Build history of the part. All positions in model axes, mm. Face numbers are marked on the shaded views. A direction names the side the tool comes from. Round coordinates to 2 decimals unless told otherwise and drop trailing zeros. Loops run counter-clockwise (first coordinate to the right, second up) from the corner with the lowest first, then second, coordinate; pieces in that order, holes last. Notation, with made-up numbers: M 31,58 L 46,58 A25 ccw 46,79 Z; hole C -36.75,87.25 d9. An arc over 180 degrees is marked long. Use one line per item in the form item = value. Start each with the question number.
Autodesk Inventor part; units mm, degrees
ref_plane "Startebene" through (0, 0, 0) normal (0, 0, 1) x (1, 0, 0)
ref_plane "Endebene" through (0, 0, 160) normal (0, 0, 1) x (1, 0, 0)
ref_plane "YZ Plane" through (0, 0, 0) normal (1, 0, 0) x (0, 1, 0)
ref_plane "Startebene" through (0, 0, 0) normal (0, 0, 1) x (1, 0, 0)
ref_plane "Endebene" through (0, 0, 160) normal (0, 0, 1) x (1, 0, 0)
sketch "Skizze" plane through (0, 0, 0) normal (0, 0, 1) x (1, 0, 0)
  line L0 (-30, -38) -> (-30, 38)
  line L1 (-18, 50) -> (18, 50)
  line L2 (30, 38) -> (30, -38)
  line L3 (18, -50) -> (-18, -50)
  arc A0 (-30, -38) -> (-18, -50) centre (-18, -38) ccw
  arc A1 (-18, 50) -> (-30, 38) centre (-18, 38) ccw
  arc A2 (30, 38) -> (18, 50) centre (18, 38) ccw
  arc A3 (18, -50) -> (30, -38) centre (18, -38) ccw
  line L4 (-14, 42) -> (14, 42)
  line L5 (22, 34) -> (22, -34)
  line L6 (14, -42) -> (-14, -42)
  line L7 (-22, -34) -> (-22, 34)
  line L8 (0, 73.4794) -> (0, -73.4794) construction
  line L9 (-45.4794, 0) -> (45.4794, 0) construction
  arc A4 (-22, -34) -> (-14, -42) centre (-14, -34) ccw
  arc A5 (-14, 42) -> (-22, 34) centre (-14, 34) ccw
  arc A6 (22, 34) -> (14, 42) centre (14, 34) ccw
  arc A7 (14, -42) -> (22, -34) centre (14, -34) ccw
  dimension "d7" = 12
  dimension "d10" = 100
  dimension "d11" = 60
  dimension "d12" = 8
  dimension "d15" = 50
  dimension "d16" = 30
  dimension "d19" = 8
  dimension "d20" = 8
extrude "Körper" add sketch "Skizze" along normal up to surface (160 mm away) from surface at 0
sketch "Sketch3" plane through (0, 0, 0) normal (0, 0, 1) x (1, 0, 0)
  line L0 (0, 0) -> (10, 0)
ref_plane "Work Plane3" through (0, 0, 0) normal (0, -1, 0) x (1, 0, 0)
sketch "Sketch4" plane through (0, 0, 0) normal (0, -1, 0) x (1, 0, 0)
  line L0 (-2, 0) -> (12, 0)
  line L1 (-2, 160) -> (12, 160)
  dimension "d18" = 160
equation "\"d7\" = G_IR"
equation "\"d10\" = G_H"
equation "\"d11\" = G_W"
equation "\"d12\" = G_T"
equation "\"d15\" = 0.5 * d10"
equation "\"d16\" = 0.5 * d11"
equation "\"d19\" = G_T"
equation "\"d20\" = G_T"
equation "\"d3\" = G_L"
equation "\"G_W\" = 60"
equation "\"G_H\" = 100"
equation "\"G_T\" = 8"
equation "\"G_IR\" = 12"
equation "\"G_L\" = d18"
equation "\"G_OFFSET_START\" = 0"
equation "\"G_OFFSET_END\" = 0"
properties part number "EN 10210-2 - 90 x 50 x 5 - 120" material "Stahl, weich"
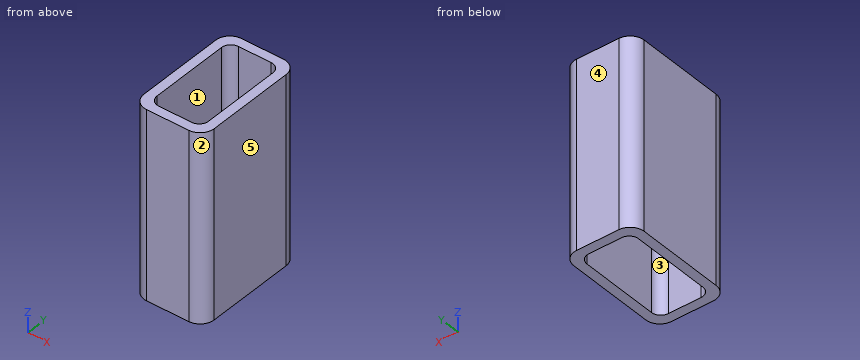
Q1. Tool access for the marked faces 1 and 2: list every direction of +Z, -Z, +X, -X, +Y, -Y with a clear straight run to the whole face (end or side of a thin tool).
Q2. Pull direction Y, two halves, no side cores. Call the marked faces 3, 4 and 5: pulls with the +Y half, pulls with the -Y half, needs draft (parallel to the pull), parting line crosses it, or undercut.
Q3. Saw through at C-C (x = -8). Give the cut face in (y, z).
Q4. Drop flat-ended pins along their axis: P1, Ø5, axis at x = -20, y = 38, coming from the -Z side; P2, Ø6, axis at x = -21.5, z = 141, coming from the -Y side. Give the stop position or say it passes through.
Q5. Saw through at B-B (y = 2). Give the cut face in (x, z), and give its area (3 significant figures).
Q6. Wall check: probe 1 along X at (y, z) = (28.5, 111.5); probe 2 along Y at (x, z) = (-11.5, 112.5); probe 3 along X at (y, z) = (39, 126.5) (3 decimals). Give the ranges that are in metal, low to high.
Q7. Saw through at A-A (z = 112.5). Give the cut face in (x, y).
Filled in:
q1.face_1 = +Z, -Z
q1.face_2 = +Z, -Z, +X, -Y
q2.face_3 = undercut
q2.face_4 = pulls with the +Y half
q2.face_5 = needs draft
q3.outline = M -50,0 L -42,0 L -42,160 L -50,160 Z; M 42,0 L 50,0 L 50,160 L 42,160 Z
q4.P1 = 0
q4.P2 = -49.99
q5.outline = M -30,0 L -22,0 L -22,160 L -30,160 Z; M 22,0 L 30,0 L 30,160 L 22,160 Z
q5.area = 2,560 mm²
q6.probe_1 = -30 to -22, 22 to 30
q6.probe_2 = -50 to -42, 42 to 50
q6.probe_3 = -29.958 to -20.245, 20.245 to 29.958
q7.outline = M -30,-38 A12 ccw -18,-50 L 18,-50 A12 ccw 30,-38 L 30,38 A12 ccw 18,50 L -18,50 A12 ccw -30,38 Z; hole M -22,-34 A8 ccw -14,-42 L 14,-42 A8 ccw 22,-34 L 22,34 A8 ccw 14,42 L -14,42 A8 ccw -22,34 Z
